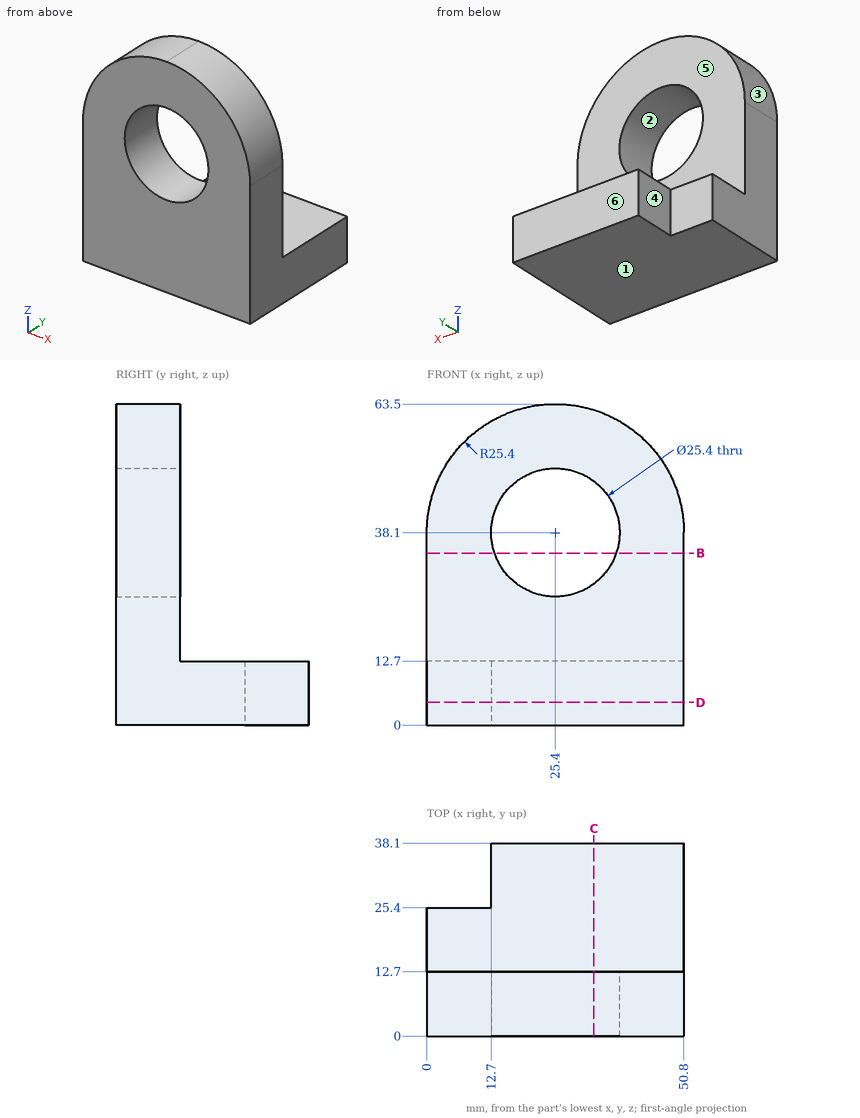
Could you check a few things on this drawing? It's one solid part, dimensions in mm from its lowest x, y, z. A direction names the side the tool comes from. Give positions to 0.01 mm unless a question says otherwise; leave off trailing zeros. Order: outer loops, then holes, each group sorted by start corner. A loop starts at its lowest first (then second) coordinate and runs counter-clockwise, first axis right, second up.
1. Suppose I cut it at B-B (z = 34). Write out the boundary of the cut face in (x, y), plus the area to 3 significant figures.
Answers below:
outline: (0, 0) - (13.38, 0) - (13.38, 12.7) - (0, 12.7) - close; (37.42, 0) - (50.8, 0) - (50.8, 12.7) - (37.42, 12.7) - close
area: 340 mm2
2. I need wall thicknesses on L1, parallel to Z at x = 25, y = 6; L2, parallel to X at y = 5, z = 38; L3, parallel to Z at x = 40.5, y = 34.5. Which ranges of each line are inside material? Lowest first, please.
Answers below:
L1: z = 0 to 25.41, 50.79 to 63.5
L2: x = 0 to 12.7, 38.1 to 50.8
L3: z = 0 to 12.7
3. Suppose I cut it at C-C (x = 33). Write out the boundary of the cut face in (y, z).
Answers below:
outline: (0, 0) - (38.1, 0) - (38.1, 12.7) - (12.7, 12.7) - (12.7, 27.93) - (0, 27.93) - close; (0, 48.27) - (12.7, 48.27) - (12.7, 62.34) - (0, 62.34) - close
4. For pin 1 (6.5 mm diameter, centred on x = 5.5, z = 5.5, fed in from +Y); pin 2 (15 mm diameter, centred on x = 25.4, z = 38.1, fed in from +Y); pin 3 (12.5 mm diameter, centred on x = 37, y = 19.5, fed in from +Z), each with a flat end and sliding along its axis, tell me the tip position at first contact or that it passes through.
Answers below:
pin 1: stops at y = 25.4
pin 2: passes through
pin 3: stops at z = 12.7
5. Thinking about a two-plate mould opening in Z: for the marked faces 1, 2 and 3, which applies, +Z half, -Z half, draft (parallel to the pull), parting line (faces both ways), or undercut?
Answers below:
face 1: -Z half
face 2: undercut
face 3: +Z half
6. Which directions (+Z, -Z, +X, -X, +Y, -Y) give clear straight access to the entire face, cutting with the end or side of a thin tool? Please do the marked faces 4, 5 and 6.
Answers below:
face 4: +Z, -Z, -X, +Y
face 5: +Z, +X, -X, +Y
face 6: +Z, -Z, +X, -X, +Y
7. Suppose I cut it at D-D (z = 4.5). Write out the boundary of the cut face in (x, y), plus the area to 3 significant figures.
Answers below:
outline: (0, 0) - (50.8, 0) - (50.8, 38.1) - (12.7, 38.1) - (12.7, 25.4) - (0, 25.4) - close
area: 1,770 mm2
